from build123d import *

# Parameters (mm, degrees)
EXTRUDE_1_DEPTH     = 30
SKETCH_2_R          = 2
CUT_EXTRUDE_1_DEPTH = 9
SKETCH_3_R          = 2
CUT_EXTRUDE_2_DEPTH = 9
SKETCH_4_R          = 1.8
CUT_EXTRUDE_3_DEPTH = 9


with BuildPart() as part:
    # 草圖1 → 填料-伸長1 (new body)
    with BuildSketch(Plane(origin=(0, 0, 0), x_dir=(1, 0, 0), z_dir=(0, 1, 0))):
        Polygon((0, 0), (0, 33.6), (-10.5, 33.6), (-10.5, 39.1), (8, 39.1), (8, 0), align=None)
    extrude(amount=EXTRUDE_1_DEPTH)

    # 草圖2 → 除料-伸長1 (cut)
    with BuildSketch(Plane(origin=(0, 0, -39.1), x_dir=(-1, 0, 0), z_dir=(0, 0, -1))):
        with Locations((4.25, 26)):
            Circle(SKETCH_2_R)
        with Locations((4.25, 18)):
            Circle(SKETCH_2_R)
        with Locations((4.25, 10)):
            Circle(SKETCH_2_R)
    extrude(amount=-CUT_EXTRUDE_1_DEPTH, mode=Mode.SUBTRACT)

    # 草圖3 → 除料-伸長2 (cut)
    with BuildSketch(Plane(origin=(8, 0, 0), x_dir=(0, 0, -1), z_dir=(1, 0, 0))):
        with Locations((14, 26)):
            Circle(SKETCH_3_R)
        with Locations((14, 18)):
            Circle(SKETCH_3_R)
        with Locations((14, 10)):
            Circle(SKETCH_3_R)
        with Locations((22, 26)):
            Circle(SKETCH_3_R)
        with Locations((22, 18)):
            Circle(SKETCH_3_R)
        with Locations((22, 10)):
            Circle(SKETCH_3_R)
    extrude(amount=-CUT_EXTRUDE_2_DEPTH, mode=Mode.SUBTRACT)

    # 草圖4 → 除料-伸長3 (cut)
    with BuildSketch(Plane.XY):
        with Locations((4, 23)):
            Circle(SKETCH_4_R)
        with Locations((4, 15)):
            Circle(SKETCH_4_R)
        with Locations((4, 7)):
            Circle(SKETCH_4_R)
    extrude(amount=-CUT_EXTRUDE_3_DEPTH, mode=Mode.SUBTRACT)


solid = part.part
Model file for the job. Use its own axes, mm. A direction names the side the tool comes from. Give positions to 0.01 mm unless a question says otherwise; leave off trailing zeros. Loops run counter-clockwise (first coordinate to the right, second up) from the corner with the lowest first, then second, coordinate; pieces in that order, holes last. Notation, with made-up numbers: (82.5, -38) -> (101.5, -38) arc R31 ccw to (101.5, -1) -> close; hole circle Ø5 at (-16.75, -27.75). An arc over 180 degrees is marked (long way). Use a Markdown table: item, result. Add a question column.
(1) Slice it at A-A on x = -4.25. List the corners of the cut face in (y, z), and give its area (3 significant figures).
(2) Wall check: line 1 along Y through (x, z) = (2, -14); line 2 along Y through (x, z) = (4, -6); line 3 along Z through (x, y) = (6.25, 17). Give the ranges that are in metal, low to high.
(3) Drop flat-ended pins along their axis: pin 1 Ø6.5 at (y, z) = (18, -14) entering from +X; pin 2 Ø15 at (y, z) = (10.5, -15) entering from -X; pin 3 Ø3 at (x, y) = (4, 7) entering from +Z. Give the stop position or say it passes through.
(4) Slice it at B-B on y = 18. List the corners of the cut face in (x, z).
(5) Slice it at D-D on z = -14. List the corners of the cut face in (x, y).
(6) Tool access for faces 1 (the cylindrical face through (4, 20, -14)), 2 (the flat face through (0, 15, -17)), 3 (the flat face through (4, 7, -9)): list every direction of +Z, -Z, +X, -X, +Y, -Y with a clear straight run to the whole face (end or side of a thin tool).
(7) Slice it at C-C on z = -35. List the corners of the cut face in (x, y), and give its area (3 significant figures).
(8) Mould opens along Y. For faces 4 (the flat face through (3, 30, -20)), 5 (the flat face through (6, 15, 0)), 6 (the cylindrical face through (-3.816, 24.048, -36.388)) say: +Y half, -Y half, draft (parallel to the pull), parting line (faces both ways), or undercut.
Filled sheet:
| question | item | result |
|---|---|---|
| 1 | outline | (0, -39.1) -> (8, -39.1) -> (8, -33.6) -> (0, -33.6) -> close; (12, -39.1) -> (16, -39.1) -> (16, -33.6) -> (12, -33.6) -> close; (20, -39.1) -> (24, -39.1) -> (24, -33.6) -> (20, -33.6) -> close; (28, -39.1) -> (30, -39.1) -> (30, -33.6) -> (28, -33.6) -> close |
| 1 | area | 99.0 mm2 |
| 2 | line 1 | 0 to 8, 12 to 16, 20 to 24, 28 to 30 |
| 2 | line 2 | 0 to 5.2, 8.8 to 13.2, 16.8 to 21.2, 24.8 to 30 |
| 2 | line 3 | -39.1 to -23.73, -20.27 to -15.73, -12.27 to 0 |
| 3 | pin 1 | x = 8 |
| 3 | pin 2 | x = 0 |
| 3 | pin 3 | z = -9 |
| 4 | outline | (-10.5, -39.1) -> (-6.25, -39.1) -> (-6.25, -33.6) -> (-10.5, -33.6) -> close; (-2.25, -39.1) -> (8, -39.1) -> (8, -24) -> (0, -24) -> (0, -33.6) -> (-2.25, -33.6) -> close; (0, -20) -> (8, -20) -> (8, -16) -> (0, -16) -> close; (0, -12) -> (8, -12) -> (8, 0) -> (0, 0) -> close |
| 5 | outline | (0, 0) -> (8, 0) -> (8, 8) -> (0, 8) -> close; (0, 12) -> (8, 12) -> (8, 16) -> (0, 16) -> close; (0, 20) -> (8, 20) -> (8, 24) -> (0, 24) -> close; (0, 28) -> (8, 28) -> (8, 30) -> (0, 30) -> close |
| 6 | face 1 | +X, -X |
| 6 | face 2 | +Z, -X, +Y, -Y |
| 6 | face 3 | +Z |
| 7 | outline | (-10.5, 0) -> (8, 0) -> (8, 30) -> (-10.5, 30) -> close; hole circle Ø4 at (-4.25, 10); hole circle Ø4 at (-4.25, 18); hole circle Ø4 at (-4.25, 26) |
| 7 | area | 517 mm2 |
| 8 | face 4 | +Y half |
| 8 | face 5 | draft |
| 8 | face 6 | undercut |
